Geometry: final body of the model. Coordinates: model frame, mm. Coordinates: 2 decimals unless noted, no trailing zeros. Order: outer loops, then holes, each group sorted by start corner. A loop starts at its lowest first (then second) coordinate and runs counter-clockwise, first axis right, second up. Notation, with made-up numbers: (-14, 25) - (16, 25) arc R25 ccw to (16, 40) - close; hole circle Ø3 at (2.5, -13.75). An arc over 180 degrees is marked (long way). Use one line per item in the form item = value. Start each with the question number.
Autodesk Inventor part; units mm, degrees
ref_plane "YZ Plane" through (0, 0, 0) normal (1, 0, 0) x (0, 1, 0)
ref_plane "XZ Plane" through (0, 0, 0) normal (0, 1, 0) x (-1, 0, 0)
ref_plane "XY Plane" through (0, 0, 0) normal (0, 0, 1) x (1, 0, 0)
sketch "Sketch1" plane through (0, 0, 0) normal (0, 0, 1) x (1, 0, 0)
  circle A0 centre (0, 0) radius 36
  circle A1 centre (0, 0) radius 65
  line L0 (45.9619, -45.9619) -> (-45.9619, 45.9619) construction
  line L1 (-45.9619, -45.9619) -> (45.9619, 45.9619) construction
  point P0 (0, 36)
  dimension "d44" = 72
  dimension "d23" = 130
extrude "Plate1" add sketch "Sketch1" along normal blind 3
sketch "Sketch6" plane through (0, 0, 0) normal (0, 0, 1) x (1, 0, 0)
  line L0 (0, 0) -> (0, 55) construction
  circle A0 centre (0, 0) radius 55 construction
  line L1 (0, 0) -> (38.8909, 38.8909) construction
  circle A1 centre (38.8909, 38.8909) radius 5.5
  dimension "d42" = 72.5
  dimension "d32" = 11
  dimension "d33" = 110
  dimension "d34" = 45
extrude "Cut2" cut sketch "Sketch6" along normal blind 3
pattern_circular "Circular Pattern2" count 4 over 360 about axis through (0, 0, -10) along (0, 0, -1) of "Cut2"
equation "\"d35\" = Thickness"
equation "\"d2\" = Thickness"
equation "\"BendRadius\" = Thickness"
equation "\"BendReliefWidth\" = Thickness"
equation "\"BendReliefDepth\" = 0.5 * Thickness"
equation "\"CornerReliefSize\" = 4 * Thickness"
equation "\"MinimumRemnant\" = 2 * Thickness"
equation "\"TransitionRadius\" = BendRadius"
equation "\"JacobiRadiusSize\" = BendRadius"
equation "\"GapSize\" = Thickness"
equation "\"Octaeder_side\" = d41"
equation "\"Octaeder_flange_lenth\" = d42"
properties part number "DSB 131 head flange"
(1) Contact query for flat-ended pins moving along their axis: pin 1 Ø1.5 at (y, z) = (-15.5, 1.5) entering from +X; pin 2 Ø1 at (x, z) = (-46.5, 0.5) entering from -Y; pin 3 Ø9 at (x, y) = (38.89, -38.89) entering from -Z. Output: stop coordinate, or through.
(2) Cut plane D-D on x = -51.5. Return the cut outline in (y, z).
(3) Material intervals for L1, parallel to X at y = 39, z = 0.1; L2, parallel to Y at x = 37.5, z = 2.45; L3, parallel to Y at x = 43.5, z = 0.3, sorted ascending. Write a range as from..to.
(4) Cut plane C-C on z = 1.15. Return the cut outline in (x, y).
(5) Draft query along Y for faces 1 (the cylindrical face through (38.17, 33.44, 1.48)), 2 (the cylindrical face through (62, -19.52, 1.48)), 3 (the flat face through (28, -28, 0)). Return one class per face: released by +Y, released by -Y, zero draft, split by the parting line, or undercut.
(6) Cut plane A-A on x = 0. Return the cut outline in (y, z), plus the area to 3 significant figures.
Check sheet entries:
q1.pin_1 = 63.3
q1.pin_2 = -45.92
q1.pin_3 = through
q2.outline = (-39.66, 0) - (39.66, 0) - (39.66, 3) - (-39.66, 3) - close
q3.L1 = -52..-44.39, -33.39..33.39, 44.39..52
q3.L2 = -53.09..-44.21, -33.57..33.57, 44.21..53.09
q3.L3 = -48.3..-41.89, -35.89..35.89, 41.89..48.3
q4.outline = circle Ø130 at (0, 0); hole circle Ø11 at (-38.89, -38.89); hole circle Ø11 at (-38.89, 38.89); hole circle Ø72 at (0, 0); hole circle Ø11 at (38.89, -38.89); hole circle Ø11 at (38.89, 38.89)
q5.face_1 = undercut
q5.face_2 = split by the parting line
q5.face_3 = zero draft
q6.outline = (-65, 0) - (-36, 0) - (-36, 3) - (-65, 3) - close; (36, 0) - (65, 0) - (65, 3) - (36, 3) - close
q6.area = 174 mm^2
